Autodesk Inventor part; units mm, degrees
ref_plane "YZ Plane" through (0, 0, 0) normal (1, 0, 0) x (0, 1, 0)
ref_plane "XZ Plane" through (0, 0, 0) normal (0, 1, 0) x (-1, 0, 0)
ref_plane "XY Plane" through (0, 0, 0) normal (0, 0, 1) x (1, 0, 0)
sketch "Boceto1" plane through (0, 0, 0) normal (0, 1, 0) x (-1, 0, 0)
  line L0 (662.5132, 1844.5674) -> (12.5132, 1844.5674)
  line L1 (12.5132, 1844.5674) -> (12.5132, 1354.5674)
  line L2 (12.5132, 1354.5674) -> (662.5132, 1354.5674)
  line L3 (662.5132, 1354.5674) -> (662.5132, 1844.5674)
  point P0 (0, 0)
  dimension "d0" = 650
  dimension "d1" = 490
extrude "Extrusión1" add sketch "Boceto1" along normal blind 5
sketch "Boceto2" plane through (0, 5, 0) normal (0, 1, 0) x (1, 0, 0)
  arc A0 (-288.7292, -1279.5674) -> (-301.2292, -1279.5674) centre (-294.9792, -1279.5674) ccw
  circle A1 centre (-548.8292, -1364.5674) radius 3
  circle A2 centre (-476.1292, -1364.5674) radius 3
  circle A3 centre (-476.1292, -1454.5674) radius 3
  circle A4 centre (-548.8292, -1454.5674) radius 3
  point P0 (0, 0)
  dimension "d6" = 6
  dimension "d7" = 253.85
  dimension "d9" = 6
  dimension "d10" = 72.7
  dimension "d11" = 6
  dimension "d12" = 6
  dimension "d13" = 90
  dimension "d14" = 90
extrude "Extrusión3" cut sketch "Boceto2" against normal through all
sketch "Boceto3" plane through (0, 5, 0) normal (0, 1, 0) x (1, 0, 0)
  line L0 (-502.9542, -1515.5674) -> (-522.0042, -1515.5674)
  line L1 (-607.4792, -1534.5674) -> (-417.4792, -1534.5674)
  line L2 (-417.4792, -1534.5674) -> (-417.4792, -1774.5674)
  line L3 (-417.4792, -1774.5674) -> (-607.4792, -1774.5674)
  line L4 (-607.4792, -1774.5674) -> (-607.4792, -1534.5674)
  line L5 (-662.5132, -1844.5674) -> (-12.5132, -1844.5674)
  point P0 (0, 0)
  point P1 (-512.4792, -1534.5674)
  point P2 (-512.4792, -1515.5674)
  dimension "d17" = 190
  dimension "d18" = 240
  dimension "d19" = 70
extrude "Extrusión4" cut sketch "Boceto3" against normal through all
properties material "Aluminio 6061"
Geometry: final body of the model. Coordinates: model frame, mm. Give positions to 0.01 mm unless a question says otherwise; leave off trailing zeros. Loops run counter-clockwise (first coordinate to the right, second up) from the corner with the lowest first, then second, coordinate; pieces in that order, holes last. Notation, with made-up numbers: (-1.75, 50) -> (22.25, 50) arc R15 ccw to (22.25, 73) -> close; hole circle Ø2 at (21.5, 46). An arc over 180 degrees is marked (long way). Return JSON: item names as keys, results as strings.
Item 1: Section C-C, the plane y = 3. Output: boundary loops of the cut face in (x, z).
Filled in:
{"outline": "(-662.51, 1354.57) -> (-12.51, 1354.57) -> (-12.51, 1844.57) -> (-662.51, 1844.57) -> close; hole (-607.48, 1534.57) -> (-417.48, 1534.57) -> (-417.48, 1774.57) -> (-607.48, 1774.57) -> close; hole circle Ø6 at (-548.83, 1364.57); hole circle Ø6 at (-548.83, 1454.57); hole circle Ø6 at (-476.13, 1364.57); hole circle Ø6 at (-476.13, 1454.57)"}
Item 2: Section B-B, the plane z = 1633.5. Output: boundary loops of the cut face in (x, y), plus the area to 3 significant figures.
Filled in:
{"outline": "(-662.51, 0) -> (-607.48, 0) -> (-607.48, 5) -> (-662.51, 5) -> close; (-417.48, 0) -> (-12.51, 0) -> (-12.51, 5) -> (-417.48, 5) -> close", "area": "2,300 mm^2"}
Item 3: Section A-A, the plane x = -441. Output: boundary loops of the cut face in (y, z).
Filled in:
{"outline": "(0, 1354.57) -> (5, 1354.57) -> (5, 1534.57) -> (0, 1534.57) -> close; (0, 1774.57) -> (5, 1774.57) -> (5, 1844.57) -> (0, 1844.57) -> close"}
Item 4: Line query: line 1 (X direction, y = 2.6, z = 1556); line 2 (Z direction, x = -431.5, y = 3.35); line 3 (X direction, y = 3.25, z = 1453). Output: solid intervals per line, ascending.
Filled in:
{"line 1": "-662.51 to -607.48, -417.48 to -12.51", "line 2": "1354.57 to 1534.57, 1774.57 to 1844.57", "line 3": "-662.51 to -551.39, -546.27 to -478.69, -473.57 to -12.51"}
